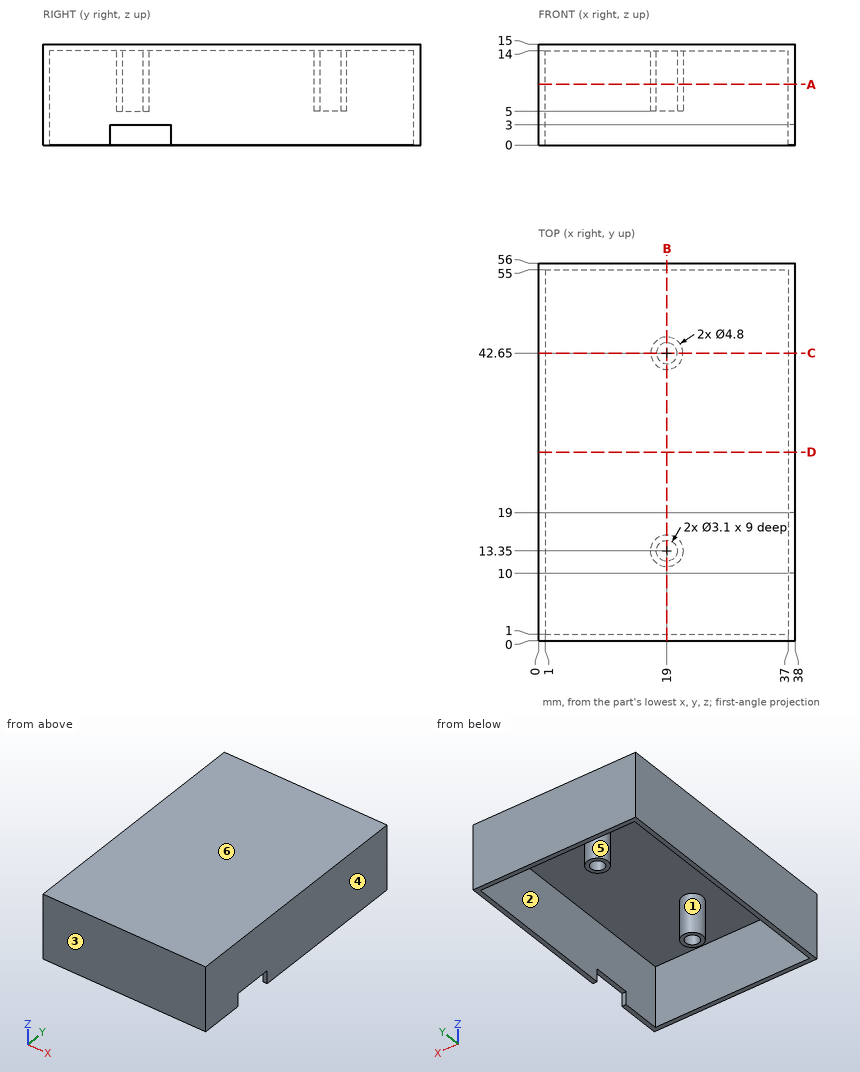
Answer from the drawing. Dimensions are ordinates in mm from the lowest x, y and z of the part. A direction names the side the tool comes from. Give positions to 0.01 mm unless a question says otherwise; leave off trailing zeros. Loops run counter-clockwise (first coordinate to the right, second up) from the corner with the lowest first, then second, coordinate; pieces in that order, holes last. Notation, with made-up numbers: (78.25, 79.5) -> (113.25, 79.5) arc R22 cw to (113.25, 110.5) -> close; hole circle Ø6 at (-13.75, 22). An arc over 180 degrees is marked (long way). One line per question, with ' | ' between items. Start each with the question number.
1) Section B-B, the plane x = 19 is taken. Determine the outline of the cut face in (y, z), then the cut area to 3 significant figures.
2) Section A-A, the plane z = 9 is taken. Determine the outline of the cut face in (x, y).
3) Section D-D, the plane y = 28 is taken. Determine the outline of the cut face in (x, z), then the cut area to 3 significant figures.
4) Section C-C, the plane y = 42.65 is taken. Determine the outline of the cut face in (x, z).
5) Straight lines are drawn through the part: L1, parallel to Y at x = 19, z = 8.25; L2, parallel to X at y = 13.35, z = 11.75; L3, parallel to Y at x = 10.5, z = 13. For each, find the intervals that lie inside material, in ascending order.
6) Each of these flat-tipped pins is pushed along its axis until it touches: pin 1 (1.1 mm diameter, centred on x = 37.5, y = 13.5, fed in from -Z); pin 2 (2.5 mm diameter, centred on x = 18.5, y = 43, fed in from -Z); pin 3 (2.5 mm diameter, centred on x = 19, y = 42.65, fed in from -Z). Where does it stop, or does it pass through?
7) Determine the mould class of the marked faces 1, 2, 3 and 4 for opening direction Y: +Y half, -Y half, draft (parallel to the pull), parting line (faces both ways), or undercut.
8) For the marked faces 5 and 6, determine the directions among +Z, -Z, +X, -X, +Y, -Y from which every point of the face is accessible in a straight line to the end or side of a thin tool.
Resolved:
1) outline: (0, 0) -> (1, 0) -> (1, 14) -> (10.95, 14) -> (10.95, 5) -> (11.8, 5) -> (11.8, 14) -> (14.9, 14) -> (14.9, 5) -> (15.75, 5) -> (15.75, 14) -> (40.25, 14) -> (40.25, 5) -> (41.1, 5) -> (41.1, 14) -> (44.2, 14) -> (44.2, 5) -> (45.05, 5) -> (45.05, 14) -> (55, 14) -> (55, 0) -> (56, 0) -> (56, 15) -> (0, 15) -> close | area: 115 mm2
2) outline: (0, 0) -> (38, 0) -> (38, 56) -> (0, 56) -> close; circle Ø4.8 at (19, 13.35); circle Ø4.8 at (19, 42.65); hole (1, 1) -> (37, 1) -> (37, 55) -> (1, 55) -> close; hole circle Ø3.1 at (19, 13.35); hole circle Ø3.1 at (19, 42.65)
3) outline: (0, 0) -> (1, 0) -> (1, 14) -> (37, 14) -> (37, 0) -> (38, 0) -> (38, 15) -> (0, 15) -> close | area: 66.0 mm2
4) outline: (0, 0) -> (1, 0) -> (1, 14) -> (16.6, 14) -> (16.6, 5) -> (17.45, 5) -> (17.45, 14) -> (20.55, 14) -> (20.55, 5) -> (21.4, 5) -> (21.4, 14) -> (37, 14) -> (37, 0) -> (38, 0) -> (38, 15) -> (0, 15) -> close
5) L1: 0 to 1, 10.95 to 11.8, 14.9 to 15.75, 40.25 to 41.1, 44.2 to 45.05, 55 to 56 | L2: 0 to 1, 16.6 to 17.45, 20.55 to 21.4, 37 to 38 | L3: 0 to 1, 55 to 56
6) pin 1: z = 3 | pin 2: z = 5 | pin 3: z = 14
7) face 1: undercut | face 2: undercut | face 3: -Y half | face 4: draft
8) face 5: -Z | face 6: +Z, +X, -X, +Y, -Y
